Input: part model. Units: mm. Frame: model coordinates. Face numbers are marked on the shaded views. A direction names the side the tool comes from. Give positions to 0.01 mm unless a question says otherwise; leave off trailing zeros. Write each loop counter-clockwise with the first axis right and the second up, starting at its lowest first coordinate (ties: lowest second). Pieces come first, ordered by that corner, then holes. Notation, with made-up numbers: (66, -28.5) -> (114, -28.5) arc R21 ccw to (114, -13.5) -> close; hole circle Ø11 at (45, 35). An arc over 180 degrees is marked (long way). Return JSON: item names as keys, results as strings. Group by question number.
Item 1: Section C-C, the plane y = 17. Return loops of the section in (x, z), then the cut area to 3 significant figures.
Item 2: Mould query, pull axis Z, two halves, no side actions, for the marked faces 1, 2 and 3. Classes: released by +Z, released by -Z, zero draft, split by the parting line, or undercut.
Item 3: Section B-B, the plane x = 10. Return loops of the section in (y, z).
Item 4: Line query: line 1 (Z direction, x = 10, y = 1.45); line 2 (Z direction, x = 5, y = 7); line 3 (Y direction, x = 4, z = 11.5). Output: solid intervals per line, ascending. Write a range as [from, to].
Item 5: Section D-D, the plane x = 26. Return loops of the section in (y, z).
Item 6: Pin query (flat end, axial travel): P1, Ø15, axis at x = 23, y = 22.5, coming from the -Z side; P2, Ø10, axis at y = 13, z = 17, coming from the +X side; P3, Ø1.5, axis at y = 19.5, z = 15, coming from the -X side; P4, Ø10, axis at x = 61.5, z = 5, coming from the +Y side. Return the tip coordinate at first contact, or that it passes through.
Item 7: Set-up query: the marked faces 4 and 5. Return all of +Z, -Z, +X, -X, +Y, -Y with unobstructed straight access to the full face (end or side cutting, diameter ignored); none if empty.
Item 8: Section A-A, the plane z = 10. Return loops of the section in (x, y).
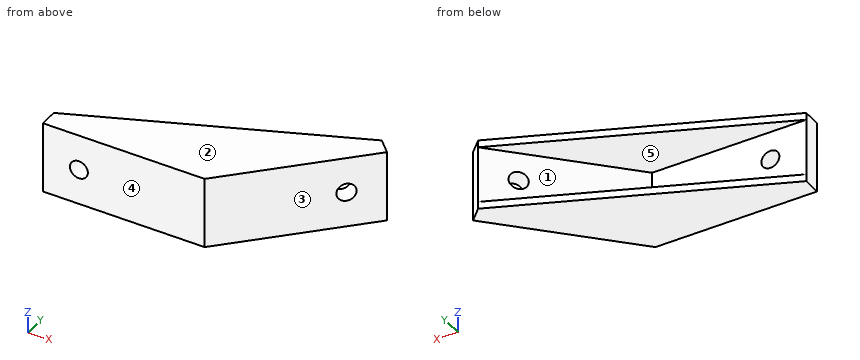
Autodesk Inventor part; units mm, degrees
ref_plane "YZ Plane" through (0, 0, 0) normal (1, 0, 0) x (0, 1, 0)
ref_plane "XZ Plane" through (0, 0, 0) normal (0, 1, 0) x (-1, 0, 0)
ref_plane "XY Plane" through (0, 0, 0) normal (0, 0, 1) x (1, 0, 0)
sketch "Sketch6" plane through (0, 0, 0) normal (0, 0, 1) x (1, 0, 0)
  line L0 (0, 0) -> (45, 0)
  line L1 (45, 0) -> (76.8198, 31.8198)
  line L2 (76.8198, 31.8198) -> (73.2843, 35.3553)
  line L3 (0, 0) -> (0, 5)
  line L4 (0, 5) -> (42.9289, 5)
  line L5 (42.9289, 5) -> (73.2843, 35.3553)
  dimension "d19" = 45
  dimension "d20" = 45
  dimension "d21" = 135
  dimension "d22" = 5
  dimension "d23" = 5
extrude "Extrusion6" add sketch "Sketch6" along normal blind 20
sketch "Sketch7" plane through (0, 0, 20) normal (0, 0, 1) x (1, 0, 0)
  line L0 (42.9289, 5) -> (0, 5)
  line L1 (76.8198, 31.8198) -> (73.2843, 35.3553)
  line L2 (0, 5) -> (73.2843, 35.3553)
  line L3 (73.2843, 35.3553) -> (42.9289, 5)
  point P0 (0, 0)
extrude "Extrusion7" add sketch "Sketch7" against normal blind 2
sketch "Sketch8" plane through (0, 0, 0) normal (0, 0, -1) x (-1, 0, 0)
  line L0 (0, 5) -> (-42.9289, 5)
  line L1 (0, 5) -> (-73.2843, 35.3553)
  line L2 (-42.9289, 5) -> (-73.2843, 35.3553)
  point P0 (0, 0)
extrude "Extrusion8" add sketch "Sketch8" against normal blind 2
sketch "Sketch9" plane through (0, 5, 18) normal (0, 1, 0) x (1, 0, 0)
  circle A0 centre (10, 8) radius 2.5
  line L0 (0, 16) -> (0, 0)
  point P0 (0, 18)
  point P1 (0, 8)
  dimension "d30" = 5
  dimension "d31" = 10
extrude "Extrusion9" cut sketch "Sketch9" against normal through all
sketch "Sketch10" plane through (42.9289, 5, 2) normal (-0.7071, 0.7071, 0) x (-0.7071, -0.7071, 0)
  circle A0 centre (-32.9289, 8) radius 2.5
  line L0 (-42.9289, 0) -> (-42.9289, 16)
  point P0 (33.8909, -2)
  point P1 (-42.9289, 8)
  dimension "d34" = 5
  dimension "d35" = 10
extrude "Extrusion10" cut sketch "Sketch10" against normal through all
properties part number "L Bracket Small"
Answer below:
{
 "1": {"outline": "(28.97, 0) -> (62, 0) -> (62, 20) -> (28.97, 20) -> (28.97, 18) -> (54.93, 18) -> (54.93, 2) -> (28.97, 2) -> close", "area": "245 mm2"},
 "2": {"face 1": "undercut", "face 2": "released by +Z", "face 3": "zero draft"},
 "3": {"outline": "(0, 0) -> (9.14, 0) -> (9.14, 2) -> (5, 2) -> (5, 7.5) -> (0, 7.5) -> close; (0, 12.5) -> (5, 12.5) -> (5, 18) -> (9.14, 18) -> (9.14, 20) -> (0, 20) -> close"},
 "4": {"line 1": "z = [0, 7.5], [12.5, 20]", "line 2": "z = [0, 2], [18, 20]", "line 3": "y = [0, 5]"},
 "5": {"outline": "(0, 0) -> (15.77, 0) -> (15.77, 2) -> (5, 2) -> (5, 18) -> (15.77, 18) -> (15.77, 20) -> (0, 20) -> close"},
 "6": {"P1": "stops at z = 0", "P2": "stops at x = 63", "P3": "stops at x = 56.68", "P4": "stops at y = 32.13"},
 "7": {"face 4": "+Z, -Z, +X, -X, -Y", "face 5": "-X, +Y"},
 "8": {"outline": "(0, 0) -> (7.5, 0) -> (7.5, 5) -> (0, 5) -> close; (12.5, 0) -> (45, 0) -> (67.98, 22.98) -> (64.45, 26.52) -> (42.93, 5) -> (12.5, 5) -> close; (67.98, 30.05) -> (71.52, 26.52) -> (76.82, 31.82) -> (73.28, 35.36) -> close"}
}
